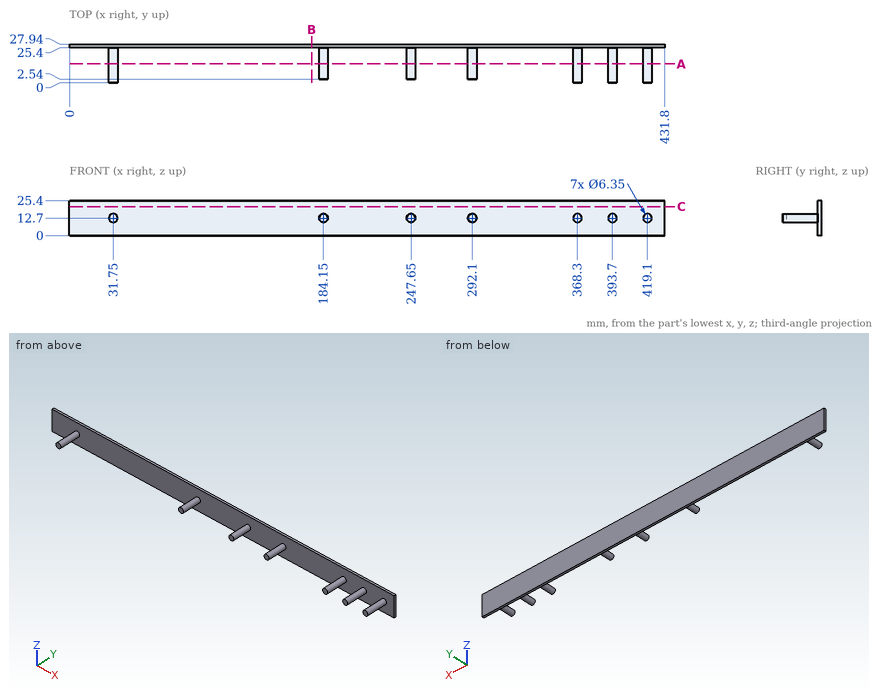
Here's the drawing with two shaded views (mm, measured from the low corner). I have some questions. Coordinates: 2 decimals unless noted, no trailing zeros. Write each loop counter-clockwise with the first axis right and the second up, starting at its lowest first coordinate (ties: lowest second). Pieces come first, ordered by that corner, then holes. Notation, with made-up numbers: M 11,84.5 L 66,84.5 A12 cw 66,96.5 Z; hole C 45,6 d10. An arc over 180 degrees is marked long. Answer as CSV lines item,"result". Start each with the question number.
1) I want a section at C-C, the plane z = 21. Please give me the cut outline in (x, y).
2) Please list where these lines run through material, in increasing order: line 1 (Y direction, x = 145, z = 19); line 2 (Z direction, x = 394, y = 13.25). Write a range as from..to.
3) For P1, Ø1, axis at y = 3, z = 15.5, coming from the -X side; P2, Ø7, axis at x = 183.5, z = 13, coming from the -Y side; P3, Ø8, axis at x = 353.5, z = 11, coming from the -Y side, each with a flat end and sliding along its axis, tell me the tip position at first contact or that it passes through.
4) I want a section at A-A, the plane y = 13.5. Please give me the cut outline in (x, z) (3 decimals), and give its area (3 significant figures).
5) I want a section at B-B, the plane x = 175.5. Please give me the cut outline in (y, z).
Data:
1,outline,"M 0,25.4 L 431.8,25.4 L 431.8,27.94 L 0,27.94 Z"
2,line 1,"y = 25.4..27.94"
2,line 2,"z = 9.54..15.86"
3,P1,"stops at x = 29.56"
3,P2,"stops at y = 2.54"
3,P3,"stops at y = 25.4"
4,outline,"C 31.75,12.7 d6.35; C 184.15,12.7 d6.35; C 247.65,12.7 d6.35; C 292.1,12.7 d6.35; C 368.3,12.7 d6.35; C 393.7,12.7 d6.35; C 419.1,12.7 d6.35"
4,area,"222 mm^2"
5,outline,"M 25.4,0 L 27.94,0 L 27.94,25.4 L 25.4,25.4 Z"
